Here's how the part is built. I have some questions about the finished solid (model axes, mm). Face numbers are marked on the shaded views. A direction names the side the tool comes from. Round coordinates to 2 decimals unless told otherwise and drop trailing zeros. Order: outer loops, then holes, each group sorted by start corner. A loop starts at its lowest first (then second) coordinate and runs counter-clockwise, first axis right, second up. Notation, with made-up numbers: M 56,35 L 94,35 A22 cw 94,44 Z; hole C 41.25,-29.75 d2. An arc over 180 degrees is marked long. Write item = value, one per line. Start each with the question number.
Item 1: I want a section at B-B, the plane z = -14. List the corners of the cut face in (x, y) for me, plus the area to 3 significant figures.
Item 2: Please list where these lines run through material, in increasing order: L1, parallel to Z at x = -40, y = -22.25; L2, parallel to X at y = -27.5, z = 11; L3, parallel to X at y = -19, z = 0.
Item 3: I'm going to push flat-ended pins straight in: P1, Ø12, axis at x = 4.5, y = -10.5, coming from the -Z side; P2, Ø22.5, axis at x = 0, z = 0, coming from the +Y side; P3, Ø24, axis at x = 41, z = 9, coming from the +Y side; P4, Ø3.5, axis at y = -6, z = -10, coming from the -X side. Where does each tip first touch, or does it pass through?
Item 4: We'd pull the mould along Z, two halves only. Please class the marked faces 4, 5, 6 and 7: pulls with the +Z half, pulls with the -Z half, needs draft (parallel to the pull), parting line crosses it, or undercut.
Item 5: I want a section at A-A, the plane x = 0. List the corners of the cut face in (y, z) for me, plus the area to 3 significant figures.
Item 6: For the marked faces 1, 2 and 3, which set-ups out of +Z, -Z, +X, -X, +Y, -Y let a thin tool reach every point of the face, with its end or its side?
Item 7: I want a section at C-C, the plane y = -4. List the corners of the cut face in (x, z) for me, plus the area to 3 significant figures.
Item 8: I want a section at D-D, the plane z = 0. List the corners of the cut face in (x, y) for me.
```python
from build123d import *

# Parameters (mm, degrees)
SKETCH1_R           = 15
BOSS_EXTRUDE2_DEPTH = 25
CUT_EXTRUDE1_REACH  = 57
SKETCH3_R           = 12.5
SKETCH3_R_2         = 5
CUT_EXTRUDE2_REACH  = 57
SKETCH5_W           = 20
SKETCH5_H           = 26
FILLET2_R           = 3
CHAMFER1_SIZE       = 2


with BuildPart() as part:
    # Sketch1 → Boss-Extrude2 (new body, symmetric)
    with BuildSketch(Plane.XY):
        with BuildLine():
            Line((-50, -30), (50, -30))
            Line((50, -30), (50, -15))
            Line((50, -15), (25, -15))
            Line((25, -15), (25, 0))
            ThreePointArc((25, 0), (0, 25), (-25, 0))
            Line((-25, 0), (-25, -15))
            Line((-25, -15), (-50, -15))
            Line((-50, -15), (-50, -30))
        make_face()
        Circle(SKETCH1_R, mode=Mode.SUBTRACT)
    extrude(amount=BOSS_EXTRUDE2_DEPTH, both=True)

    # Sketch3 → Cut-Extrude1 (cut, up to next)
    with BuildSketch(Plane.XZ.offset(30), mode=Mode.PRIVATE) as cut_extrude1_sk1:
        Circle(SKETCH3_R)
    cut_extrude1_tool1 = extrude(cut_extrude1_sk1.sketch, amount=-CUT_EXTRUDE1_REACH, mode=Mode.PRIVATE) & part.part
    add(cut_extrude1_tool1.solids().sort_by_distance((0, -30, 0))[0], mode=Mode.SUBTRACT)
    # Sketch3 → Cut-Extrude1 (cut, up to next)
    with BuildSketch(Plane.XZ.offset(30), mode=Mode.PRIVATE) as cut_extrude1_sk2:
        with Locations((-40, 15)):
            Circle(SKETCH3_R_2)
    cut_extrude1_tool2 = extrude(cut_extrude1_sk2.sketch, amount=-CUT_EXTRUDE1_REACH, mode=Mode.PRIVATE) & part.part
    add(cut_extrude1_tool2.solids().sort_by_distance((-40, -30, 15))[0], mode=Mode.SUBTRACT)
    # Sketch3 → Cut-Extrude1 (cut, up to next)
    with BuildSketch(Plane.XZ.offset(30), mode=Mode.PRIVATE) as cut_extrude1_sk3:
        with Locations((-40, -15)):
            Circle(SKETCH3_R_2)
    cut_extrude1_tool3 = extrude(cut_extrude1_sk3.sketch, amount=-CUT_EXTRUDE1_REACH, mode=Mode.PRIVATE) & part.part
    add(cut_extrude1_tool3.solids().sort_by_distance((-40, -30, -15))[0], mode=Mode.SUBTRACT)

    # Sketch5 → Cut-Extrude2 (cut, up to next)
    with BuildSketch(Plane.XZ.offset(30), mode=Mode.PRIVATE) as cut_extrude2_sk1:
        with Locations((40, 0)):
            Rectangle(SKETCH5_W, SKETCH5_H)
    cut_extrude2_tool1 = extrude(cut_extrude2_sk1.sketch, amount=-CUT_EXTRUDE2_REACH, mode=Mode.PRIVATE) & part.part
    add(cut_extrude2_tool1.solids().sort_by_distance((40, -30, 0))[0], mode=Mode.SUBTRACT)

    # Fillet2
    fillet2_edges = [part.edges().sort_by_distance(p)[0] for p in [
        (-25, -15, 0),
        (25, -15, 0),
        (30, -22.5, -13),
        (30, -22.5, 13),
    ]]
    fillet(fillet2_edges, radius=FILLET2_R)

    # Chamfer1
    chamfer1_edges = [part.edges().sort_by_distance(p)[0] for p in [
        (50, -22.5, -25),
        (-50, -22.5, -25),
        (50, -22.5, 25),
        (50, -22.5, 13),
        (50, -22.5, -13),
        (-50, -22.5, 25),
    ]]
    chamfer(chamfer1_edges, length=CHAMFER1_SIZE)


solid = part.part
```
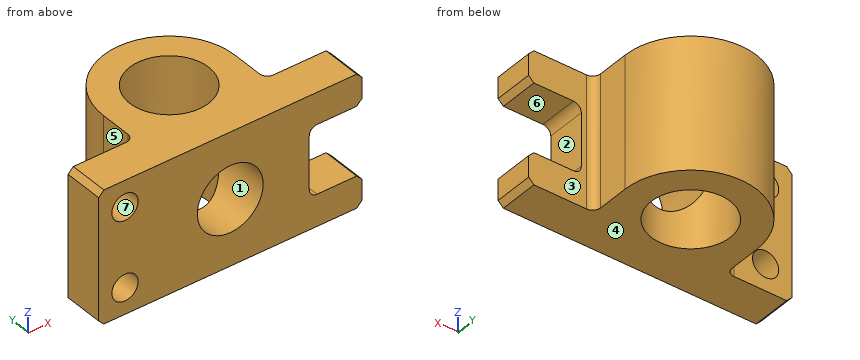
Filled in:
q1.outline = M -50,-30 L -44.9,-30 L -44.9,-15 L -50,-15 Z; M -35.1,-30 L 49,-30 L 49,-15 L 28,-15 A3 cw 25,-12 L 25,0 A25 ccw -25,0 L -25,-12 A3 cw -28,-15 L -35.1,-15 Z; hole C 0,0 d30
q1.area = 2,370 mm^2
q2.L1 = -25 to -20, -10 to 10, 20 to 25
q2.L2 = -50 to -43, -37 to -5.94, 5.94 to 30.17
q2.L3 = -50 to -12.5, 12.5 to 30
q3.P1 = -25
q3.P2 = 25
q3.P3 = -15
q3.P4 = -25
q4.face_4 = pulls with the -Z half
q4.face_5 = needs draft
q4.face_6 = undercut
q4.face_7 = undercut
q5.outline = M -30,-25 L -15,-25 L -15,-12.5 L -30,-12.5 Z; M -30,12.5 L -15,12.5 L -15,25 L -30,25 Z; M 15,-25 L 25,-25 L 25,25 L 15,25 Z
q5.area = 875 mm^2
q6.face_1 = -Y
q6.face_2 = +X, +Y, -Y
q6.face_3 = +Z, -Z, +X, +Y
q7.outline = M -25,-25 L -14.46,-25 L -14.46,25 L -25,25 Z; M 14.46,-25 L 25,-25 L 25,25 L 14.46,25 Z
q7.area = 1,050 mm^2
q8.outline = M -50,-30 L -12.5,-30 L -12.5,-8.29 A15 cw long 12.5,-8.29 L 12.5,-30 L 30,-30 L 30,-15 L 28,-15 A3 cw 25,-12 L 25,0 A25 ccw -25,0 L -25,-12 A3 cw -28,-15 L -50,-15 Z
